Read the model definition and answer for the solid it produces. Units are mm, in the model's axes. Coordinates: 2 decimals unless noted, no trailing zeros. Order: outer loops, then holes, each group sorted by start corner. A loop starts at its lowest first (then second) coordinate and runs counter-clockwise, first axis right, second up. Notation, with made-up numbers: (79, 20.25) - (106, 20.25) arc R36 ccw to (106, 59.25) - close; hole circle Ø1 at (-14.5, -31). An arc over 180 degrees is marked (long way). Use one line per item in the form item = value.
Autodesk Inventor part; units mm, degrees
ref_plane "YZ Plane" through (0, 0, 0) normal (1, 0, 0) x (0, 1, 0)
ref_plane "XZ Plane" through (0, 0, 0) normal (0, 1, 0) x (-1, 0, 0)
ref_plane "XY Plane" through (0, 0, 0) normal (0, 0, 1) x (1, 0, 0)
sketch "スケッチ1" plane through (0, 0, 0) normal (0, 0, 1) x (1, 0, 0)
  line L0 (0, 3.1754) -> (2.75, 1.5877)
  line L1 (2.75, 1.5877) -> (2.75, -1.5877)
  line L2 (2.75, -1.5877) -> (0, -3.1754)
  line L3 (0, -3.1754) -> (-2.75, -1.5877)
  line L4 (-2.75, -1.5877) -> (-2.75, 1.5877)
  line L5 (-2.75, 1.5877) -> (0, 3.1754)
  point P0 (0, 0)
  point P1 (0, 0)
  dimension "d0" = 5.5
extrude "押し出し1" add sketch "スケッチ1" along normal blind 40
sketch "スケッチ2" plane through (0, 0, 40) normal (0, 0, 1) x (1, 0, 0)
  point P0 (0, 0)
hole "穴1" at (0, 0, 40) direction (0, 0, -1) diameter 2.459 end through all
properties part number "ジュラコンスペーサー（六角）_AS-340B" material "アセタール樹脂、黒"
(1) Section D-D, the plane y = 2 is taken. Write down the section's boundary in (x, z).
Answer list:
outline = (-2.04, 0) - (2.04, 0) - (2.04, 40) - (-2.04, 40) - close
(2) Section A-A, the plane y = 0 is taken. Write down the section's boundary in (x, z), then the cut area to 3 significant figures.
Answer list:
outline = (-2.75, 0) - (-1.23, 0) - (-1.23, 40) - (-2.75, 40) - close; (1.23, 0) - (2.75, 0) - (2.75, 40) - (1.23, 40) - close
area = 122 mm2
(3) The mould has two halves that part along X. Classify faces 1 (the cylindrical face through (0.748, 0.976, 19.72)), 2 (the flat face through (-1.36, -2.39, 19.72)), 3 (the flat face through (0, -1.4, 40)): +X half, -X half, draft (parallel to the pull), parting line (faces both ways), or undercut.
Answer list:
face_1 = undercut
face_2 = -X half
face_3 = draft
(4) Section B-B, the plane z = 11 is taken. Write down the section's boundary in (x, y), then the cut area to 3 significant figures.
Answer list:
outline = (-2.75, -1.59) - (0, -3.18) - (2.75, -1.59) - (2.75, 1.59) - (0, 3.18) - (-2.75, 1.59) - close; hole circle Ø2.46 at (0, 0)
area = 21.4 mm2
(5) Section C-C, the plane x = -0.5 is taken. Write down the section's boundary in (y, z), then the cut area to 3 significant figures.
Answer list:
outline = (-2.89, 0) - (-1.12, 0) - (-1.12, 40) - (-2.89, 40) - close; (1.12, 0) - (2.89, 0) - (2.89, 40) - (1.12, 40) - close
area = 141 mm2
(6) Straight lines are drawn through the part: L1, parallel to X at y = 0, z = 25.5; L2, parallel to X at y = 1, z = 17; L3, parallel to Y at x = 0.7, z = 11. For each, find the intervals that lie inside material, in ascending order.
Answer list:
L1 = -2.75 to -1.23, 1.23 to 2.75
L2 = -2.75 to -0.72, 0.72 to 2.75
L3 = -2.77 to -1.01, 1.01 to 2.77
